Here's how the part is built. I have some questions about the finished solid (model axes, mm). A direction names the side the tool comes from. Coordinates: 2 decimals unless noted, no trailing zeros. Write each loop counter-clockwise with the first axis right and the second up, starting at its lowest first coordinate (ties: lowest second). Pieces come first, ordered by that corner, then holes.
Item 1: If we section it at A-A (y = 0): Please give me the cut outline in (x, z) (3 decimals), then the cut area to 3 significant figures.
Item 2: If we section it at D-D (z = 3.75): Please give me the cut outline in (x, y) (3 decimals), then the cut area to 3 significant figures.
Item 3: If I drill on line 1 (Y direction, x = 0, z = 1.5) (3 decimals); line 2 (Y direction, x = 0, z = 5); line 3 (Z direction, x = -3, y = 1.5), over which ranges is the centre line in solid material (lowest first)?
Item 4: I'm going to push flat-ended pins straight in: pin 1 Ø1.5 at (x, z) = (2.5, 5) entering from +Y; pin 2 Ø2 at (y, z) = (-2.5, 4.5) entering from +X; pin 3 Ø3 at (x, z) = (2.5, 1) entering from -Y. Where does each tip first touch, or does it pass through?
Item 5: If we section it at C-C (z = 5.75): Please give me the cut outline in (x, y), then the cut area to 3 significant figures.
Item 6: For faces 1 (the face through (1, -3, 6.9)), 2 (the face through (-0.4, 3.04, 2.42)), which set-ups out of +Z, -Z, +X, -X, +Y, -Y let a thin tool reach every point of the face, with its end or its side?
Item 7: We'd pull the mould along Y, two halves only. Please class faces 3 (the face through (-0.54, -2.44, 3.24)), 4 (the face through (-1.08, -4.88, 5.64)), 5 (the face through (-0.1, -3.3, 4.9)): +Y half, -Y half, draft (parallel to the pull), parting line (faces both ways), or undercut.
from build123d import *

# Parameters (mm, degrees)
SKETCH1_R           = 3.065
BOSS_EXTRUDE1_DEPTH = 4.9
SKETCH2_R           = 5
BOSS_EXTRUDE2_DEPTH = 2
SKETCH3_R           = 2.5
CUT_EXTRUDE1_DEPTH  = 7.9
CHAMFER1_SIZE       = 0.5
CHAMFER2_SIZE       = 0.5


with BuildPart() as part:
    # Sketch1 → Boss-Extrude1 (new body)
    with BuildSketch(Plane.XY):
        Circle(SKETCH1_R)
    extrude(amount=BOSS_EXTRUDE1_DEPTH)

    # Sketch2 → Boss-Extrude2 (add)
    with BuildSketch(Plane.XY.offset(4.9)):
        Circle(SKETCH2_R)
    extrude(amount=BOSS_EXTRUDE2_DEPTH)

    # Sketch3 → Cut-Extrude1 (cut, through all)
    with BuildSketch(Plane.XY.offset(6.9)):
        Circle(SKETCH3_R)
    extrude(amount=-CUT_EXTRUDE1_DEPTH, mode=Mode.SUBTRACT)

    # Chamfer1
    chamfer1_edges = [part.edges().sort_by_distance(p)[0] for p in [
        (-5, 0, 6.9),
    ]]
    chamfer(chamfer1_edges, length=CHAMFER1_SIZE)

    # Chamfer2
    chamfer2_edges = [part.edges().sort_by_distance(p)[0] for p in [
        (-2.5, 0, 6.9),
    ]]
    chamfer(chamfer2_edges, length=CHAMFER2_SIZE)


solid = part.part
Answer list:
1. outline: (-5, 4.9) - (-3.065, 4.9) - (-3.065, 0) - (-2.5, 0) - (-2.5, 6.4) - (-3, 6.9) - (-4.5, 6.9) - (-5, 6.4) - close; (2.5, 0) - (3.065, 0) - (3.065, 4.9) - (5, 4.9) - (5, 6.4) - (4.5, 6.9) - (3, 6.9) - (2.5, 6.4) - close
1. area: 15.0 mm2
2. outline: circle Ø6.13 at (0, 0); hole circle Ø5 at (0, 0)
2. area: 9.88 mm2
3. line 1: y = -3.065 to -2.5, 2.5 to 3.065
3. line 2: y = -5 to -2.5, 2.5 to 5
3. line 3: z = 4.9 to 6.9
4. pin 1: stops at y = 4.68
4. pin 2: stops at x = 4.74
4. pin 3: stops at y = -2.9
5. outline: circle Ø10 at (0, 0); hole circle Ø5 at (0, 0)
5. area: 58.9 mm2
6. face 1: +Z, +X, -X, +Y, -Y
6. face 2: -Z
7. face 3: undercut
7. face 4: parting line
7. face 5: draft
